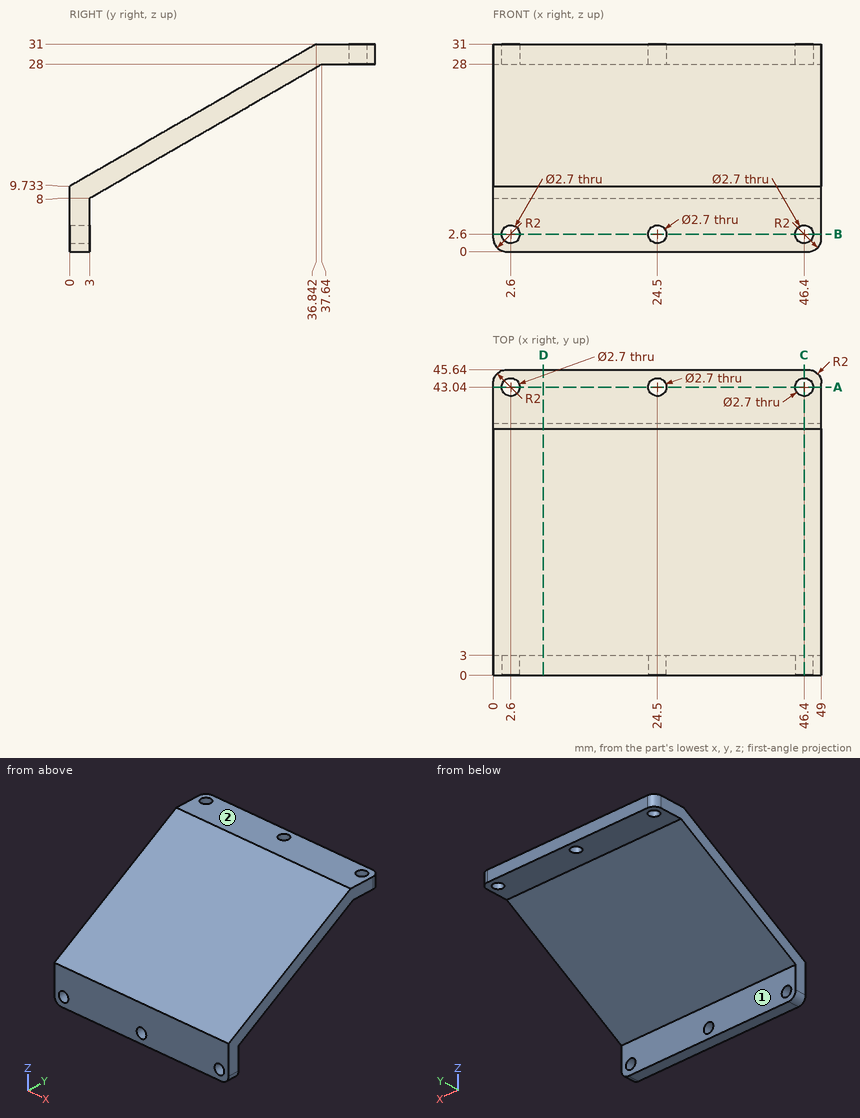
Print and shaded views of the part. All mm, measured from the part's lowest x, y and z. A direction names the side the tool comes from. Coordinates: 2 decimals unless noted, no trailing zeros. Order: outer loops, then holes, each group sorted by start corner. A loop starts at its lowest first (then second) coordinate and runs counter-clockwise, first axis right, second up.
(1) Slice it at B-B, the plane z = 2.6. Write the cut outline in (x, y).
Check sheet entries:
outline: (0, 0) - (1.25, 0) - (1.25, 3) - (0, 3) - close; (3.95, 0) - (23.15, 0) - (23.15, 3) - (3.95, 3) - close; (25.85, 0) - (45.05, 0) - (45.05, 3) - (25.85, 3) - close; (47.75, 0) - (49, 0) - (49, 3) - (47.75, 3) - close
(2) Slice it at A-A, the plane y = 43.04. Write the cut outline in (x, z), and give its area (3 significant figures).
Check sheet entries:
outline: (0, 28) - (1.25, 28) - (1.25, 31) - (0, 31) - close; (3.95, 28) - (23.15, 28) - (23.15, 31) - (3.95, 31) - close; (25.85, 28) - (45.05, 28) - (45.05, 31) - (25.85, 31) - close; (47.75, 28) - (49, 28) - (49, 31) - (47.75, 31) - close
area: 123 mm2
(3) Tool access for the marked faces 1 and 2: list every direction of +Z, -Z, +X, -X, +Y, -Y with a clear straight run to the whole face (end or side of a thin tool).
Check sheet entries:
face 1: -Z, +X, -X, +Y
face 2: +Z, +X, -X, +Y, -Y
(4) Pin check, flat tips, straight feed: pin 1 Ø1.5 at (x, y) = (5.5, 7) entering from +Z; pin 2 Ø12 at (x, y) = (35.5, 20.5) entering from +Z; pin 3 Ø12 at (x, y) = (30.5, 12.5) entering from -Z. Stop position of each tip, or through.
Check sheet entries:
pin 1: stops at z = 14.21
pin 2: stops at z = 25.03
pin 3: stops at z = 10.02
(5) Slice it at C-C, the plane x = 46.4. Write the cut outline in (y, z), and give its area (3 significant figures).
Check sheet entries:
outline: (0, 0) - (3, 0) - (3, 1.25) - (0, 1.25) - close; (0, 3.95) - (3, 3.95) - (3, 8) - (37.64, 28) - (41.69, 28) - (41.69, 31) - (36.84, 31) - (0, 9.73) - close; (44.39, 28) - (45.64, 28) - (45.64, 31) - (44.39, 31) - close
area: 159 mm2
(6) Probe L1, parallel to Y at x = 21, z = 4; L2, parallel to Y at x = 24, z = 29 (1 decimal); L3, parallel to Z at x = 24.5, y = 1.95. List the from-to ranges inside material, lowest first.
Check sheet entries:
L1: y = 0 to 3
L2: y = 33.4 to 41.8, 44.3 to 45.6
L3: z = 0 to 1.25, 3.95 to 10.86
(7) Slice it at D-D, the plane x = 7.5. Write the cut outline in (y, z).
Check sheet entries:
outline: (0, 0) - (3, 0) - (3, 8) - (37.64, 28) - (45.64, 28) - (45.64, 31) - (36.84, 31) - (0, 9.73) - close
